```python
from build123d import *

# Parameters (mm, degrees)
BOSS_EXTRU_1_DEPTH      = 32
ESQUISSE2_R             = 11
BOSS_EXTRU_2_DEPTH      = 2
BOSS_EXTRU_3_DEPTH      = 22
ESQUISSE4_R             = 1.25
ENL_V_MAT_EXTRU_1_DEPTH = 10


with BuildPart() as part:
    # Esquisse1 → Boss.-Extru.1 (new body)
    with BuildSketch(Plane.XY):
        Polygon((21.15, 18.15), (18.15, 21.15), (-18.15, 21.15), (-21.15, 18.15), (-21.15, -18.15), (-18.15, -21.15), (18.15, -21.15), (21.15, -18.15), align=None)
    extrude(amount=BOSS_EXTRU_1_DEPTH)

    # Esquisse2 → Boss.-Extru.2 (add)
    with BuildSketch(Plane.XY.offset(32)):
        Circle(ESQUISSE2_R)
    extrude(amount=BOSS_EXTRU_2_DEPTH)

    # Esquisse3 → Boss.-Extru.3 (add)
    with BuildSketch(Plane.XY.offset(34)):
        with BuildLine():
            Line((-2, 1.5), (2, 1.5))
            ThreePointArc((2, 1.5), (0, -2.5), (-2, 1.5))
        make_face()
    extrude(amount=BOSS_EXTRU_3_DEPTH)

    # Esquisse4 → Enlèv. mat.-Extru.1 (cut)
    with BuildSketch(Plane.XY.offset(32)):
        with Locations((-15.5, 15.5)):
            Circle(ESQUISSE4_R)
        with Locations((15.5, 15.5)):
            Circle(ESQUISSE4_R)
        with Locations((15.5, -15.5)):
            Circle(ESQUISSE4_R)
        with Locations((-15.5, -15.5)):
            Circle(ESQUISSE4_R)
    extrude(amount=-ENL_V_MAT_EXTRU_1_DEPTH, mode=Mode.SUBTRACT)


solid = part.part
```
CAD build for the part. Positions are in the model's coordinates, mm. A direction names the side the tool comes from. Round coordinates to 2 decimals unless told otherwise and drop trailing zeros. Write each loop counter-clockwise with the first axis right and the second up, starting at its lowest first coordinate (ties: lowest second). Pieces come first, ordered by that corner, then holes. Notation, with made-up numbers: (47, 69) - (85, 69) arc R36 cw to (85, 108) - close; hole circle Ø7 at (65.25, 23.5). An arc over 180 degrees is marked (long way). Write item = value, one per line. Start each with the question number.
Q1. Band-saw the part on A-A (z = 29). Give the cut face in (x, y), then the cut area to 3 significant figures.
Q2. Band-saw the part on B-B (y = 0). Give the cut face in (x, z).
Q3. Mould opens along Y. For faces 1 (the cylindrical face through (-2.38, -10.74, 32.99)), 2 (the flat face through (-3, 0, 34)), 3 (the cylindrical face through (15.34, -14.26, 27.07)), 4 (the flat face through (-16, 16, 22)) say: pulls with the +Y half, pulls with the -Y half, needs draft (parallel to the pull), parting line crosses it, or undercut.
Q4. Band-saw the part on D-D (z = 37). Give the cut face in (x, y), then the cut area to 3 significant figures.
Q5. Drop flat-ended pins along their axis: pin 1 (2 mm diameter, centred on x = -16, y = 15.5, fed in from +Z); pin 2 (2 mm diameter, centred on x = -15.5, y = -15.5, fed in from +Z); pin 3 (3 mm diameter, centred on x = 15.5, y = -15.5, fed in from -Z); pin 4 (3 mm diameter, centred on x = 1.5, z = 50, fed in from -Y). Give the stop position or say it passes through.
Q6. Band-saw the part on C-C (x = 15.5). Give the cut face in (y, z), then the cut area to 3 significant figures.
Q7. Probe L1, parallel to Y at x = -15.5, z = 27.75; L2, parallel to X at y = 16, z = 31.5. List the from-to ranges inside material, lowest first. Write a range as from..to.
Q8. Which spindle directions (+Z, -Z, +X, -X, +Y, -Y) get a long thin tool onto all of the face, cutting with end or side? Do faces 5 (the flat face through (21.15, 0, 16)), 6 (the cylindrical face through (0.1, -2.5, 44.8)), 7 (the flat face through (0, 1.5, 45)). Say none if no direction does.
Answers below:
q1.outline = (-21.15, -18.15) - (-18.15, -21.15) - (18.15, -21.15) - (21.15, -18.15) - (21.15, 18.15) - (18.15, 21.15) - (-18.15, 21.15) - (-21.15, 18.15) - close; hole circle Ø2.5 at (-15.5, -15.5); hole circle Ø2.5 at (-15.5, 15.5); hole circle Ø2.5 at (15.5, -15.5); hole circle Ø2.5 at (15.5, 15.5)
q1.area = 1,750 mm2
q2.outline = (-21.15, 0) - (21.15, 0) - (21.15, 32) - (11, 32) - (11, 34) - (2.5, 34) - (2.5, 56) - (-2.5, 56) - (-2.5, 34) - (-11, 34) - (-11, 32) - (-21.15, 32) - close
q3.face_1 = parting line crosses it
q3.face_2 = needs draft
q3.face_3 = undercut
q3.face_4 = undercut
q4.outline = (-2, 1.5) arc R2.5 ccw (long way) to (2, 1.5) - close
q4.area = 16.8 mm2
q5.pin_1 = 32
q5.pin_2 = 22
q5.pin_3 = 0
q5.pin_4 = -2.5
q6.outline = (-21.15, 0) - (21.15, 0) - (21.15, 32) - (16.75, 32) - (16.75, 22) - (14.25, 22) - (14.25, 32) - (-14.25, 32) - (-14.25, 22) - (-16.75, 22) - (-16.75, 32) - (-21.15, 32) - close
q6.area = 1,300 mm2
q7.L1 = -21.15..-16.75, -14.25..14.25, 16.75..21.15
q7.L2 = -21.15..-16.65, -14.35..14.35, 16.65..21.15
q8.face_5 = +Z, -Z, +X, +Y, -Y
q8.face_6 = +Z
q8.face_7 = +Z, +X, -X, +Y
